Verification items for this drawing (mm, ordinates from the low corner). Round coordinates to 2 decimals unless told otherwise and drop trailing zeros. Order: outer loops, then holes, each group sorted by start corner. A loop starts at its lowest first (then second) coordinate and runs counter-clockwise, first axis right, second up. Notation, with made-up numbers: (77.5, 22) -> (95.5, 22) arc R17 cw to (95.5, 31) -> close; hole circle Ø3 at (51, -30). An arc over 180 degrees is marked (long way). Answer in a Markdown table with one row per item. Add a question column.
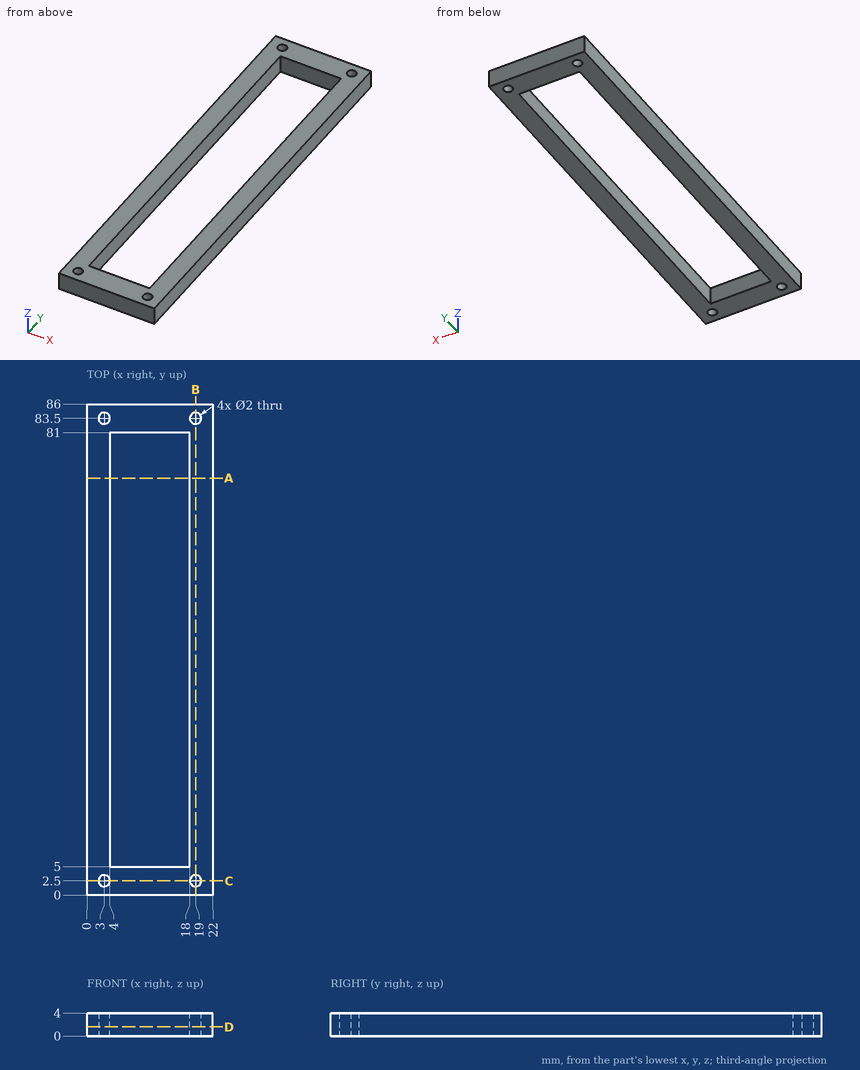
1) Thickness scan on L1, parallel to Y at x = 3, z = 3.05; L2, parallel to X at y = 83.5, z = 1.6; L3, parallel to Y at x = 16.25, z = 1.55. Record the ranges inside material, lowest first. Write a range as [from, to].
2) Cross-section at A-A, the plane y = 73. Record the boundary of the cut face in (x, z), and give its area (3 significant figures).
3) Cross-section at D-D, the plane z = 1.6. Record the boundary of the cut face in (x, y).
4) Cross-section at B-B, the plane x = 19. Record the boundary of the cut face in (y, z).
5) Cross-section at C-C, the plane y = 2.5. Record the boundary of the cut face in (x, z), and give its area (3 significant figures).
6) Depth check by flat-ended pin: P1, Ø1.8, axis at x = 3, y = 83.5, coming from the -Z side. Enter the tip coordinate at first touch or a pass-through.
Results below:
| question | item | result |
|---|---|---|
| 1 | L1 | [0, 1.5], [3.5, 82.5], [84.5, 86] |
| 1 | L2 | [0, 2], [4, 18], [20, 22] |
| 1 | L3 | [0, 5], [81, 86] |
| 2 | outline | (0, 0) -> (4, 0) -> (4, 4) -> (0, 4) -> close; (18, 0) -> (22, 0) -> (22, 4) -> (18, 4) -> close |
| 2 | area | 32.0 mm² |
| 3 | outline | (0, 0) -> (22, 0) -> (22, 86) -> (0, 86) -> close; hole circle Ø2 at (3, 2.5); hole circle Ø2 at (3, 83.5); hole (4, 5) -> (18, 5) -> (18, 81) -> (4, 81) -> close; hole circle Ø2 at (19, 2.5); hole circle Ø2 at (19, 83.5) |
| 4 | outline | (0, 0) -> (1.5, 0) -> (1.5, 4) -> (0, 4) -> close; (3.5, 0) -> (82.5, 0) -> (82.5, 4) -> (3.5, 4) -> close; (84.5, 0) -> (86, 0) -> (86, 4) -> (84.5, 4) -> close |
| 5 | outline | (0, 0) -> (2, 0) -> (2, 4) -> (0, 4) -> close; (4, 0) -> (18, 0) -> (18, 4) -> (4, 4) -> close; (20, 0) -> (22, 0) -> (22, 4) -> (20, 4) -> close |
| 5 | area | 72.0 mm² |
| 6 | P1 | through |
